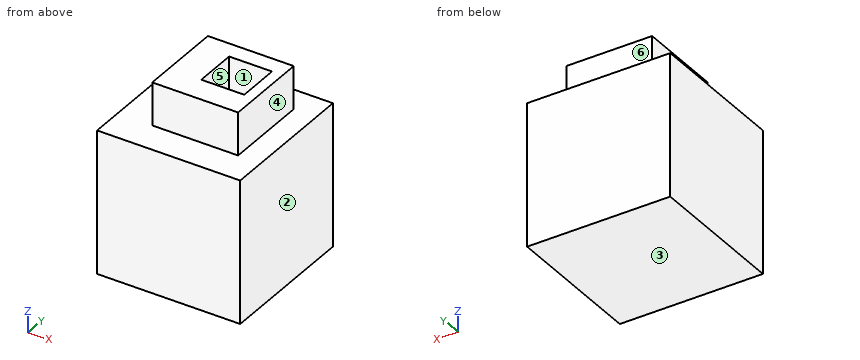
```python
from build123d import *

# Parameters (mm, degrees)
F0_W     = 50
F0_H     = 50
F1_DEPTH = 50
F2_W     = 30
F2_H     = 30
F2_W_2   = 15
F2_H_2   = 15
F3_DEPTH = 15
F4_DEPTH = 15


with BuildPart() as f1:
    # F0 (on Top) → F1 (new body)
    with BuildSketch(Plane.XY):
        with Locations((-25, 25)):
            Rectangle(F0_W, F0_H)
    extrude(amount=F1_DEPTH)

    # F2 (on face) → F3 (join)
    with BuildSketch(Plane.XY.offset(50)):
        with Locations((-22.896898, 26.06651)):
            Rectangle(F2_W, F2_H)
        with Locations((-19.131815, 27.618613)):
            Rectangle(F2_W_2, F2_H_2, mode=Mode.SUBTRACT)
    extrude(amount=F3_DEPTH)

    # F2 (on face) → F4 (join)
    with BuildSketch(Plane.XY.offset(50)):
        with Locations((-22.896898, 26.06651)):
            Rectangle(F2_W, F2_H)
        with Locations((-19.131815, 27.618613)):
            Rectangle(F2_W_2, F2_H_2, mode=Mode.SUBTRACT)
    extrude(amount=F4_DEPTH)


solid = f1.part
```
Can you work these out from the model? Positions are in its coordinate system, mm. Face numbers are marked on the shaded views. A direction names the side the tool comes from. Coordinates: 2 decimals unless noted, no trailing zeros. Loops run counter-clockwise (first coordinate to the right, second up) from the corner with the lowest first, then second, coordinate; pieces in that order, holes last. Notation, with made-up numbers: M -13.5,59.5 L 10.5,59.5 A18 cw 10.5,73.5 Z; hole C -21.5,29.25 d9. An arc over 180 degrees is marked long. Put each result on its own line as item: value. Start each with the question number.
(1) Imagine slicing it at A-A on z = 52. List the corners of the cut face in (x, y) for me, and give its area (3 significant figures).
(2) I need wall thicknesses on probe 1 along Y at (x, z) = (-16.5, 55); probe 2 along Z at (x, y) = (-40, 23.5); probe 3 along X at (y, z) = (38, 60.5). Which ranges of each line are inside material? Lowest first, please.
(3) Imagine slicing it at B-B on y = 22. List the corners of the cut face in (x, z) for me.
(4) Which directions (+Z, -Z, +X, -X, +Y, -Y) give clear straight access to the entire face, cutting with the end or side of a thin tool? Please do the marked faces 4, 5 and 6.
(5) We'd pull the mould along X, two halves only. Please class the marked faces 1, 2 and 3: +X half, -X half, draft (parallel to the pull), parting line (faces both ways), or undercut.
(6) Will these pins go through, and if not, where does the flat tip stop? pin 1 Ø2 at (x, y) = (-11.5, 9.5) entering from -Z; pin 2 Ø7.5 at (x, z) = (-24.5, 59) entering from +Y; pin 3 Ø4.5 at (y, z) = (27.5, 60) entering from -X; pin 4 Ø4.5 at (y, z) = (33, 59) entering from +X.
(7) Imagine slicing it at D-D on y = 37. List the corners of the cut face in (x, z) for me, and give its area (3 significant figures).
(8) Imagine slicing it at C-C on x = -20. List the corners of the cut face in (y, z) for me.
Worked answers:
1. outline: M -37.9,11.07 L -7.9,11.07 L -7.9,41.07 L -37.9,41.07 Z; hole M -26.63,20.12 L -11.63,20.12 L -11.63,35.12 L -26.63,35.12 Z
1. area: 675 mm2
2. probe 1: y = 11.07 to 20.12, 35.12 to 41.07
2. probe 2: z = 0 to 50
2. probe 3: x = -37.9 to -7.9
3. outline: M -50,0 L 0,0 L 0,50 L -7.9,50 L -7.9,65 L -11.63,65 L -11.63,50 L -26.63,50 L -26.63,65 L -37.9,65 L -37.9,50 L -50,50 Z
4. face 4: +Z, +X, +Y, -Y
4. face 5: +Z
4. face 6: +Z, +X, -X, +Y
5. face 1: undercut
5. face 2: +X half
5. face 3: draft
6. pin 1: stops at z = 0
6. pin 2: stops at y = 41.07
6. pin 3: stops at x = -37.9
6. pin 4: stops at x = -7.9
7. outline: M -50,0 L 0,0 L 0,50 L -7.9,50 L -7.9,65 L -37.9,65 L -37.9,50 L -50,50 Z
7. area: 2,950 mm2
8. outline: M 0,0 L 50,0 L 50,50 L 41.07,50 L 41.07,65 L 35.12,65 L 35.12,50 L 20.12,50 L 20.12,65 L 11.07,65 L 11.07,50 L 0,50 Z
